Source: CAD feature listing. Evaluate the final solid. Frame: model axes, mm. Face numbers are marked on the shaded views. Coordinates: 2 decimals unless noted, no trailing zeros. Loops run counter-clockwise (first coordinate to the right, second up) from the corner with the lowest first, then second, coordinate; pieces in that order, holes last.
Item 1: Pin query (flat end, axial travel): pin 1 Ø2 at (y, z) = (-4.5, -54.5) entering from -X; pin 2 Ø2 at (x, y) = (-29, -4.5) entering from -Z; pin 3 Ø1.2 at (y, z) = (-1.5, -2.5) entering from -X; pin 4 Ø1.6 at (x, y) = (-15.5, -5) entering from -Z. Return the tip coordinate at first contact, or that it passes through.
Item 2: Pull-direction query (Z, two-part tool) for the marked faces 1 and 2; classes: +Z half, -Z half, draft (parallel to the pull), parting line (faces both ways), or undercut.
Item 3: Section query A-A, the plane x = 10. Return the cut outline in (y, z), then the cut area to 3 significant figures.
Item 4: Line query: probe 1 along Z at (x, y) = (-36, -3.25); probe 2 along X at (y, z) = (-1.5, -10.5); probe 3 along Z at (x, y) = (-11, -4.45). Output: solid intervals per line, ascending.
Item 5: Section query C-C, the plane y = -1.95. Return the cut outline in (x, z), then the cut area to 3 significant figures.
Item 6: Section query B-B, the plane z = -5. Return the cut outline in (x, y), then the cut area to 3 significant figures.
Item 7: Section query D-D, the plane x = -105. Return the cut outline in (y, z), then the cut area to 3 significant figures.
```python
from build123d import *

# Parameters (mm, degrees)
F1_DEPTH = 6
F2_DEPTH = 4
F3_DEPTH = 4
F4_DEPTH = 4


# Not quite as in the source:
# - a feature names something its author has since deleted; it is built from what else it names


with BuildPart() as f1:
    # F0 (on Front) → F1 (new body)
    with BuildSketch(Plane.XZ):
        with BuildLine():
            Line((-100.5, 195), (-100.5, -195))
            Line((-100.5, -195), (-40.5, -195))
            Line((-40.5, -195), (40.5, -195))
            ThreePointArc((40.5, -195), (82.9264068712, -177.4264068712), (100.5, -135))
            Line((100.5, -135), (100.5, 157))
            ThreePointArc((100.5, 157), (89.3700576851, 183.8700576851), (62.5, 195))
            Line((62.5, 195), (-100.5, 195))
        make_face()
        with BuildLine():
            Line((96.5, 157), (96.5, -135))
            ThreePointArc((96.5, -135), (80.0979797464, -174.5979797464), (40.5, -191))
            Line((40.5, -191), (-90.5, -191))
            ThreePointArc((-90.5, -191), (-94.7426406871, -189.2426406871), (-96.5, -185))
            Line((-96.5, -185), (-96.5, 185))
            ThreePointArc((-96.5, 185), (-94.7426406871, 189.2426406871), (-90.5, 191))
            Line((-90.5, 191), (62.5, 191))
            ThreePointArc((62.5, 191), (86.5416305603, 181.0416305603), (96.5, 157))
        make_face(mode=Mode.SUBTRACT)
        with BuildLine():
            ThreePointArc((-142.7480761254, -193.9473684211), (-143.3275959396, -194.3693704052), (-143.8526478713, -194.8574783429))
            ThreePointArc((-143.8526478713, -194.8574783429), (-143.2065526025, -194.9642631589), (-142.552668078, -195))
            Line((-142.552668078, -195), (-100.5, -195))
            Line((-100.5, -195), (-100.5, 195))
            Line((-100.5, 195), (-123.66718427, 195))
            ThreePointArc((-123.66718427, 195), (-123.8241029609, 194.9979476927), (-123.9809143034, 194.9917921748))
            ThreePointArc((-123.9809143034, 194.9917921748), (-123.7745554417, 194.7731997599), (-123.5575071568, 194.5652173913))
            ThreePointArc((-123.5575071568, 194.5652173913), (-113.9097026951, 181.1601405667), (-110.5, 165))
            Line((-110.5, 165), (-110.5, -135))
            ThreePointArc((-110.5, -135), (-119.0889477731, -168.5958727285), (-142.7480761254, -193.9473684211))
        make_face()
        with BuildLine():
            ThreePointArc((-146.0024255254, -184.0909090909), (-148.4365234746, -190.1748385726), (-143.8526478713, -194.8574783429))
            ThreePointArc((-143.8526478713, -194.8574783429), (-143.3275959396, -194.3693704052), (-142.7480761254, -193.9473684211))
            ThreePointArc((-142.7480761254, -193.9473684211), (-119.0889477731, -168.5958727285), (-110.5, -135))
            Line((-110.5, -135), (-110.5, 165))
            ThreePointArc((-110.5, 165), (-113.9097026951, 181.1601405667), (-123.5575071568, 194.5652173913))
            ThreePointArc((-123.5575071568, 194.5652173913), (-123.7745554417, 194.7731997599), (-123.9809143034, 194.9917921748))
            ThreePointArc((-123.9809143034, 194.9917921748), (-129.2065981407, 191.3054053807), (-128.139320225, 185))
            ThreePointArc((-128.139320225, 185), (-122.4748292311, 175.7046626932), (-120.5, 165))
            Line((-120.5, 165), (-120.5, -135))
            ThreePointArc((-120.5, -135), (-127.2559652709, -162.6599487665), (-146.0024255254, -184.0909090909))
        make_face()
        with BuildLine():
            ThreePointArc((40.5, -191), (80.0979797464, -174.5979797464), (96.5, -135))
            Line((96.5, -135), (96.5, 157))
            ThreePointArc((96.5, 157), (86.5416305603, 181.0416305603), (62.5, 191))
            Line((62.5, 191), (-90.5, 191))
            ThreePointArc((-90.5, 191), (-94.7426406871, 189.2426406871), (-96.5, 185))
            Line((-96.5, 185), (-96.5, -185))
            ThreePointArc((-96.5, -185), (-94.7426406871, -189.2426406871), (-90.5, -191))
            Line((-90.5, -191), (40.5, -191))
        make_face()
        with BuildLine():
            Line((86.5, 135), (86.5, -135))
            ThreePointArc((86.5, -135), (73.0269119346, -167.5269119346), (40.5, -181))
            Line((40.5, -181), (-40.5, -181))
            ThreePointArc((-40.5, -181), (-73.0269119346, -167.5269119346), (-86.5, -135))
            Line((-86.5, -135), (-86.5, 135))
            ThreePointArc((-86.5, 135), (-73.0269119346, 167.5269119346), (-40.5, 181))
            Line((-40.5, 181), (40.5, 181))
            ThreePointArc((40.5, 181), (73.0269119346, 167.5269119346), (86.5, 135))
        make_face(mode=Mode.SUBTRACT)
    extrude(amount=F1_DEPTH)

    # F0 (on Front) → F2 (join)
    with BuildSketch(Plane.XZ):
        with BuildLine():
            Line((-110.5, -205), (40.5, -205))
            ThreePointArc((40.5, -205), (89.9974746831, -184.4974746831), (110.5, -135))
            Line((110.5, -135), (110.5, 165))
            ThreePointArc((110.5, 165), (98.7842712475, 193.2842712475), (70.5, 205))
            Line((70.5, 205), (-110.5, 205))
            Line((-110.5, 205), (-119.5161332303, 205))
            ThreePointArc((-119.5161332303, 205), (-124.9956061498, 201.4444583295), (-123.9809143034, 194.9917921748))
            ThreePointArc((-123.9809143034, 194.9917921748), (-123.8241029609, 194.9979476927), (-123.66718427, 195))
            Line((-123.66718427, 195), (-100.5, 195))
            Line((-100.5, 195), (62.5, 195))
            ThreePointArc((62.5, 195), (89.3700576851, 183.8700576851), (100.5, 157))
            Line((100.5, 157), (100.5, -135))
            ThreePointArc((100.5, -135), (82.9264068712, -177.4264068712), (40.5, -195))
            Line((40.5, -195), (-40.5, -195))
            Line((-40.5, -195), (-100.5, -195))
            Line((-100.5, -195), (-142.552668078, -195))
            ThreePointArc((-142.552668078, -195), (-143.2065526025, -194.9642631589), (-143.8526478713, -194.8574783429))
            ThreePointArc((-143.8526478713, -194.8574783429), (-145.0283155871, -201.3606005652), (-139.5121969362, -205))
            Line((-139.5121969362, -205), (-110.5, -205))
        make_face()
    extrude(amount=F2_DEPTH)

    # F0 (on Front) → F3 (cut)
    with BuildSketch(Plane.XZ):
        with BuildLine():
            ThreePointArc((-146.0024255254, -184.0909090909), (-148.4365234746, -190.1748385726), (-143.8526478713, -194.8574783429))
            ThreePointArc((-143.8526478713, -194.8574783429), (-143.3275959396, -194.3693704052), (-142.7480761254, -193.9473684211))
            ThreePointArc((-142.7480761254, -193.9473684211), (-119.0889477731, -168.5958727285), (-110.5, -135))
            Line((-110.5, -135), (-110.5, 165))
            ThreePointArc((-110.5, 165), (-113.9097026951, 181.1601405667), (-123.5575071568, 194.5652173913))
            ThreePointArc((-123.5575071568, 194.5652173913), (-123.7745554417, 194.7731997599), (-123.9809143034, 194.9917921748))
            ThreePointArc((-123.9809143034, 194.9917921748), (-129.2065981407, 191.3054053807), (-128.139320225, 185))
            ThreePointArc((-128.139320225, 185), (-122.4748292311, 175.7046626932), (-120.5, 165))
            Line((-120.5, 165), (-120.5, -135))
            ThreePointArc((-120.5, -135), (-127.2559652709, -162.6599487665), (-146.0024255254, -184.0909090909))
        make_face()
    extrude(amount=F3_DEPTH, mode=Mode.SUBTRACT)

    # F0 (on Front) → F4 (cut)
    with BuildSketch(Plane.XZ):
        with BuildLine():
            ThreePointArc((40.5, -191), (80.0979797464, -174.5979797464), (96.5, -135))
            Line((96.5, -135), (96.5, 157))
            ThreePointArc((96.5, 157), (86.5416305603, 181.0416305603), (62.5, 191))
            Line((62.5, 191), (-90.5, 191))
            ThreePointArc((-90.5, 191), (-94.7426406871, 189.2426406871), (-96.5, 185))
            Line((-96.5, 185), (-96.5, -185))
            ThreePointArc((-96.5, -185), (-94.7426406871, -189.2426406871), (-90.5, -191))
            Line((-90.5, -191), (40.5, -191))
        make_face()
        with BuildLine():
            Line((86.5, 135), (86.5, -135))
            ThreePointArc((86.5, -135), (73.0269119346, -167.5269119346), (40.5, -181))
            Line((40.5, -181), (-40.5, -181))
            ThreePointArc((-40.5, -181), (-73.0269119346, -167.5269119346), (-86.5, -135))
            Line((-86.5, -135), (-86.5, 135))
            ThreePointArc((-86.5, 135), (-73.0269119346, 167.5269119346), (-40.5, 181))
            Line((-40.5, 181), (40.5, 181))
            ThreePointArc((40.5, 181), (73.0269119346, 167.5269119346), (86.5, 135))
        make_face(mode=Mode.SUBTRACT)
    extrude(amount=F4_DEPTH, mode=Mode.SUBTRACT)


solid = f1.part
```
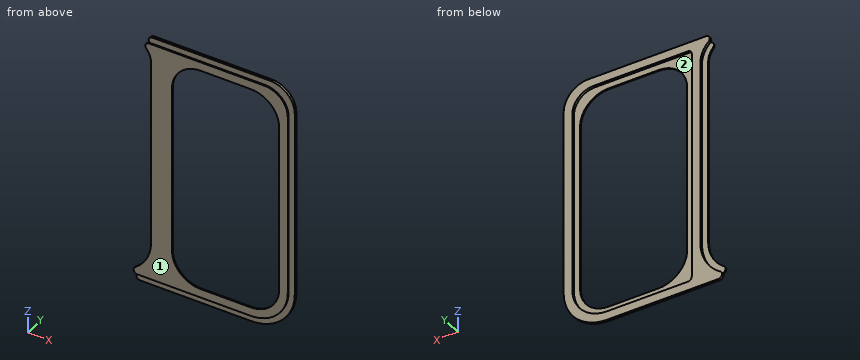
Verdict:
1. pin 1: stops at x = -120.5
1. pin 2: stops at z = -205
1. pin 3: stops at x = -110.5
1. pin 4: stops at z = -195
2. face 1: draft
2. face 2: undercut
3. outline: (-6, -195) - (-4, -195) - (-4, -205) - (0, -205) - (0, -191) - (-4, -191) - (-4, -181) - (-6, -181) - close; (-6, 181) - (-4, 181) - (-4, 191) - (0, 191) - (0, 205) - (-4, 205) - (-4, 195) - (-6, 195) - close
3. area: 168 mm2
4. probe 1: z = -205 to -191, 191 to 205
4. probe 2: x = -110.5 to -96.5, 96.5 to 110.5
4. probe 3: z = -195 to -181, 181 to 195
5. outline: (-142.75, -193.95) arc R6 ccw to (-139.51, -205) - (40.5, -205) arc R70 ccw to (110.5, -135) - (110.5, 165) arc R40 ccw to (70.5, 205) - (-119.52, 205) arc R6 ccw to (-123.56, 194.57) arc R40 cw to (-110.5, 165) - (-110.5, -135) arc R70 cw to start; hole (-96.5, -185) arc R6 ccw to (-90.5, -191) - (40.5, -191) arc R56 ccw to (96.5, -135) - (96.5, 157) arc R34 ccw to (62.5, 191) - (-90.5, 191) arc R6 ccw to (-96.5, 185) - close
5. area: 17,600 mm2
6. outline: (-120.5, -6) - (-86.5, -6) - (-86.5, -4) - (-96.5, -4) - (-96.5, 0) - (-110.5, 0) - (-110.5, -4) - (-120.5, -4) - close; (86.5, -6) - (100.5, -6) - (100.5, -4) - (110.5, -4) - (110.5, 0) - (96.5, 0) - (96.5, -4) - (86.5, -4) - close
6. area: 208 mm2
7. outline: (-6, -195) - (-4, -195) - (-4, -205) - (0, -205) - (0, 205) - (-4, 205) - (-4, 195) - (-6, 195) - close
7. area: 2,420 mm2
